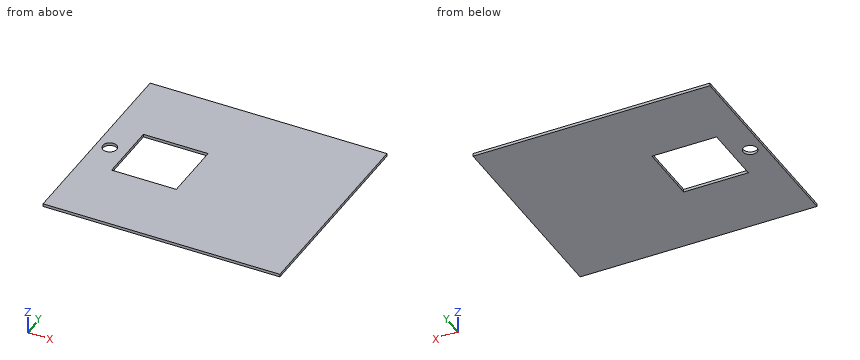
from build123d import *

# Parameters (mm, degrees)
SKETCH1_W           = 250
SKETCH1_H           = 220
BOSS_EXTRUDE1_DEPTH = 3
SKETCH2_W           = 68.242640687
SKETCH2_H           = 65.242640687
CUT_EXTRUDE1_DEPTH  = 3
SKETCH3_R           = 7.392015443
CUT_EXTRUDE2_DEPTH  = 10


with BuildPart() as part:
    # Sketch1 → Boss-Extrude1 (new body)
    with BuildSketch(Plane.XY):
        with Locations((28.200067517, 87.906622336)):
            Rectangle(SKETCH1_W, SKETCH1_H)
    extrude(amount=BOSS_EXTRUDE1_DEPTH)

    # Sketch2 → Cut-Extrude1 (cut)
    with BuildSketch(Plane(origin=(0, 0, 0), x_dir=(-1, 0, 0), z_dir=(0, 0, -1))):
        with Locations((30.322878983, 88.52794268)):
            Rectangle(SKETCH2_W, SKETCH2_H)
    extrude(amount=-CUT_EXTRUDE1_DEPTH, mode=Mode.SUBTRACT)

    # Sketch3 → Cut-Extrude2 (cut)
    with BuildSketch(Plane(origin=(0, 0, 0), x_dir=(-1, 0, 0), z_dir=(0, 0, -1))):
        with Locations((82.764080487, 87.906622336)):
            Circle(SKETCH3_R)
    extrude(amount=-CUT_EXTRUDE2_DEPTH, mode=Mode.SUBTRACT)


solid = part.part
Build history of the part. All positions in model axes, mm. Give positions to 0.01 mm unless a question says otherwise; leave off trailing zeros. Order: outer loops, then holes, each group sorted by start corner. A loop starts at its lowest first (then second) coordinate and runs counter-clockwise, first axis right, second up. Notation, with made-up numbers: M 79.5,2.25 L 93.5,2.25 A9 cw 93.5,7.25 Z; hole C 21,-9 d4. An arc over 180 degrees is marked long. Put each result on its own line as item: value.
Item 1: Slice it at C-C, the plane z = 0.6. Write the cut outline in (x, y).
From the geometry:
outline: M -96.8,-22.09 L 153.2,-22.09 L 153.2,197.91 L -96.8,197.91 Z; hole C -82.76,87.91 d14.78; hole M -64.44,55.91 L 3.8,55.91 L 3.8,121.15 L -64.44,121.15 Z
Item 2: Slice it at B-B, the plane x = -15. Write the cut outline in (y, z), plus the area to 3 significant figures.
From the geometry:
outline: M -22.09,0 L 55.91,0 L 55.91,3 L -22.09,3 Z; M 121.15,0 L 197.91,0 L 197.91,3 L 121.15,3 Z
area: 464 mm2
Item 3: Probe line 1 (X direction, y = 114, z = 1.6); line 2 (X direction, y = 89.5, z = 1.75); line 3 (Y direction, x = -7.5, z = 0.55). List the from-to ranges inside material, lowest first. Write a range as [from, to].
From the geometry:
line 1: x = [-96.8, -64.44], [3.8, 153.2]
line 2: x = [-96.8, -89.98], [-75.55, -64.44], [3.8, 153.2]
line 3: y = [-22.09, 55.91], [121.15, 197.91]
Item 4: Slice it at A-A, the plane y = 67.5. Write the cut outline in (x, z).
From the geometry:
outline: M -96.8,0 L -64.44,0 L -64.44,3 L -96.8,3 Z; M 3.8,0 L 153.2,0 L 153.2,3 L 3.8,3 Z
